Part model, mm, in its own coordinate system. A direction names the side the tool comes from. Round coordinates to 2 decimals unless told otherwise and drop trailing zeros. Write each loop counter-clockwise with the first axis right and the second up, starting at its lowest first coordinate (ties: lowest second). Pieces come first, ordered by that corner, then holes. Notation, with made-up numbers: (-28, 1) -> (-18, 1) arc R23 cw to (-18, 34) -> close; hole circle Ø3 at (-26, 45.5). An arc over 180 degrees is marked (long way). Return JSON: item names as keys, results as strings. Group by question number.
```python
from build123d import *

# Parameters (mm, degrees)
SKETCH2_R           = 15
BOSS_EXTRUDE2_DEPTH = 130
SKETCH5_R           = 11
BOSS_EXTRUDE3_DEPTH = 35
CHAMFER1_SIZE       = 2


with BuildPart() as part:
    # Sketch2 → Boss-Extrude2 (new body)
    with BuildSketch(Plane.XY):
        Circle(SKETCH2_R)
    extrude(amount=BOSS_EXTRUDE2_DEPTH)

    # Sketch4 → Revolve1 (revolve)
    with BuildSketch(Plane(origin=(0, 0, 0), x_dir=(0, 0, -1), z_dir=(1, 0, 0))):
        Polygon((-130, 0), (-172.3, 0), (-172.3, 14), (-133, 14), (-130, 15), align=None)
    revolve(axis=Axis((0, 0, 130), (0, 0, 1)))

    # Sketch5 → Boss-Extrude3 (add, symmetric)
    with BuildSketch(Plane(origin=(0, 0, 0), x_dir=(0, 0, -1), z_dir=(1, 0, 0))):
        with Locations((-158.3, 0)):
            Circle(SKETCH5_R)
    extrude(amount=BOSS_EXTRUDE3_DEPTH, both=True)

    # Chamfer1
    chamfer1_edges = [part.edges().sort_by_distance(p)[0] for p in [
        (0, -14, 172.3),
    ]]
    chamfer(chamfer1_edges, length=CHAMFER1_SIZE)


solid = part.part
```
Item 1: Cut at A-A (z = 158.3). Write the cut outline in (x, y).
Item 2: Cut at C-C (y = 0). Write the cut outline in (x, z).
Item 3: Wall check: L1, parallel to X at y = -1, z = 83.5; L2, parallel to Y at x = 11, z = 149; L3, parallel to X at y = 0.25, z = 146. Give the ranges that are in metal, low to high.
Item 4: Cut at D-D (z = 15). Write the cut outline in (x, y).
Item 5: Flat gauge pins, fed straight in: P1, Ø8, axis at y = 8.5, z = 107.5, coming from the -X side; P2, Ø1.5, axis at x = 11.5, z = 61, coming from the -Y side; P3, Ø1.5, axis at x = 9, z = 44.5, coming from the +Y side. Where does each tip first touch, or does it go through?
Item 6: Two-plate mould, pull along Z, no slides. Class faces 4 (the face through (-4.224, 13.413, 132.812)), 5 (the face through (0, 0, 0)), 6 (the face through (0, 0, 172.3)), 7 (the face through (13.67, -3.03, 147.24)): released by +Z, released by -Z, zero draft, split by the parting line, or undercut.
Item 7: Which spindle directions (+Z, -Z, +X, -X, +Y, -Y) get a long thin tool onto all of the face, cutting with end or side? Do faces 1 (the face through (-24.57, 0.48, 169.29)), 2 (the face through (22.01, -6.69, 167.03)), 3 (the face through (-14.985, 0.66, 64.09)). Say none if no direction does.
Item 8: Cut at B-B (x = 0). Write the cut outline in (y, z), then the cut area to 3 significant figures.
Checks:
{
 "1": {"outline": "(-35, -11) -> (-8.66, -11) arc R14 ccw to (8.66, -11) -> (35, -11) -> (35, 11) -> (8.66, 11) arc R14 ccw to (-8.66, 11) -> (-35, 11) -> close"},
 "2": {"outline": "(-35, 147.3) -> (-14, 147.3) -> (-14, 133) -> (-15, 130) -> (-15, 0) -> (15, 0) -> (15, 130) -> (14, 133) -> (14, 147.3) -> (35, 147.3) -> (35, 169.3) -> (14, 169.3) -> (14, 170.3) -> (12, 172.3) -> (-12, 172.3) -> (-14, 170.3) -> (-14, 169.3) -> (-35, 169.3) -> close"},
 "3": {"L1": "x = -14.97 to 14.97", "L2": "y = -8.66 to 8.66", "L3": "x = -14 to 14"},
 "4": {"outline": "circle Ø30 at (0, 0)"},
 "5": {"P1": "stops at x = -14.31", "P2": "stops at y = -10.46", "P3": "stops at y = 12.53"},
 "6": {"face 4": "undercut", "face 5": "released by -Z", "face 6": "released by +Z", "face 7": "undercut"},
 "7": {"face 1": "-X", "face 2": "+X", "face 3": "-Z"},
 "8": {"outline": "(-15, 0) -> (15, 0) -> (15, 130) -> (14, 133) -> (14, 170.3) -> (12, 172.3) -> (-12, 172.3) -> (-14, 170.3) -> (-14, 133) -> (-15, 130) -> close", "area": "5,080 mm2"}
}
